from build123d import *

# Parameters (mm, degrees)
F0_W     = 900
F0_H     = 750
F1_DEPTH = 25.4
F3_DEPTH = 914.4
F5_DEPTH = 25.4


with BuildPart() as f1:
    # F0 (on Top) → F1 (new body)
    with BuildSketch(Plane.XY):
        Rectangle(F0_W, F0_H)
    extrude(amount=F1_DEPTH)

    # F2 (on face) → F3 (join)
    with BuildSketch(Plane(origin=(0, 0, 0), x_dir=(1, 0, 0), z_dir=(0, 0, -1))):
        Polygon((-424.6, 375), (-450, 375), (-450, -375), (-424.6, -361.6), align=None)
        Polygon((-424.6, -361.6), (-450, -375), (450, -375), (424.6, -361.6), align=None)
        Polygon((424.6, -361.6), (450, -375), (450, 375), (424.6, 375), align=None)
    extrude(amount=F3_DEPTH)

    # F4 (on face) → F5 (cut)
    with BuildSketch(Plane.XZ.offset(-361.6)):
        Polygon((424.6, -137.324512), (-424.6, -164.4), (-424.6, -914.4), (424.6, -914.4), align=None)
    extrude(amount=-F5_DEPTH, mode=Mode.SUBTRACT)


solid = f1.part
Work out the finished part from the listing and answer in its coordinate system (mm). A direction names the side the tool comes from. Coordinates: 2 decimals unless noted, no trailing zeros. Write each loop counter-clockwise with the first axis right and the second up, starting at its lowest first coordinate (ties: lowest second). Pieces come first, ordered by that corner, then holes. Notation, with made-up numbers: M -23,-16.5 L 14,-16.5 A13 ccw 14,7.5 Z; hole C 32.5,26 d2. An arc over 180 degrees is marked long. Write item = value, one per line.
1. The part is cut by section C-C (z = -61). Determine the outline of the cut face in (x, y).
Solution:
outline = M -450,-375 L -424.6,-375 L -424.6,361.6 L 424.6,361.6 L 424.6,-375 L 450,-375 L 450,375 L -450,375 Z
2. The part is cut by section D-D (x = -359.5). Determine the outline of the cut face in (y, z).
Solution:
outline = M -375,0 L 361.6,0 L 361.6,-162.32 L 375,-162.32 L 375,25.4 L -375,25.4 Z
3. A flat-ended cylindrical pin translates along its axis: pin 1 (12 mm diameter, centred on x = 311, y = -217.5, fed in from -Z). Find the tip coordinate at first contact, or state that the pin passes through.
Solution:
pin_1 = 0
4. For faces 1 (the face through (2, -375, 10)), 2 (the face through (-6, -2, 0)), determine the directions among +Z, -Z, +X, -X, +Y, -Y from which every point of the face is accessible in a straight line to the end or side of a thin tool.
Solution:
face_1 = +Z, -Z, +X, -X, -Y
face_2 = -Z, -Y
5. The part is cut by section B-B (y = 320). Determine the outline of the cut face in (x, z).
Solution:
outline = M -450,-914.4 L -424.6,-914.4 L -424.6,0 L 424.6,0 L 424.6,-914.4 L 450,-914.4 L 450,25.4 L -450,25.4 Z
6. Straight lines are drawn through the part: line 1 (X direction, y = 17.5, z = -762); line 2 (Z direction, x = -91.5, y = -331); line 3 (Y direction, x = -405.5, z = -17). For each, find the intervals that lie inside material, in ascending order. Write a range as from..to.
Solution:
line_1 = -450..-424.6, 424.6..450
line_2 = 0..25.4
line_3 = 361.6..375
7. The part is cut by section A-A (z = -454). Determine the outline of the cut face in (x, y), then the cut area to 3 significant figures.
Solution:
outline = M -450,-375 L -424.6,-375 L -424.6,375 L -450,375 Z; M 424.6,-375 L 450,-375 L 450,375 L 424.6,375 Z
area = 38,100 mm2
8. Determine the mould class of faces 3 (the face through (-450, -5, -438)), 4 (the face through (424.6, -5, -451)), 5 (the face through (-6, 5, 25.4)), 6 (the face through (450, -5, -451)) for opening direction X: released by +X, released by -X, zero draft, split by the parting line, or undercut.
Solution:
face_3 = released by -X
face_4 = undercut
face_5 = zero draft
face_6 = released by +X
